Build history of the part. All positions in model axes, mm. A direction names the side the tool comes from. Round coordinates to 2 decimals unless told otherwise and drop trailing zeros. Write each loop counter-clockwise with the first axis right and the second up, starting at its lowest first coordinate (ties: lowest second). Pieces come first, ordered by that corner, then holes.
Item 1: Band-saw the part on A-A, the plane x = 226. Write the cut outline in (y, z).
Item 2: Drop flat-ended pins along their axis: pin 1 Ø2 at (y, z) = (152.5, 74) entering from +X; pin 2 Ø5 at (x, z) = (255.5, 34.5) entering from -Y; pin 3 Ø5 at (x, z) = (257, 33) entering from +Y. Give the stop position or say it passes through.
Item 3: Band-saw the part on D-D, the plane y = 128.5. Write the cut outline in (x, z), then the cut area to 3 significant figures.
Item 4: Wall check: probe 1 along X at (y, z) = (92.5, 76); probe 2 along Y at (x, z) = (237.5, 63); probe 3 along X at (y, z) = (147, 58). Give the ranges that are in metal, low to high.
Item 5: 3-axis set-ups, long thin cutter, end or side, ignore diameter. For faces 1 (the flat face through (256, 102.8, 49)), 2 (the flat face through (234, 82.8, 49)), 3 (the cylindrical face through (214.423, 88.583, 49.3)): which of +Z, -Z, +X, -X, +Y, -Y reach the whole face in a straight line?
Item 6: Band-saw the part on C-C, the plane z = 15. Write the cut outline in (x, y).
Item 7: Mould opens along X. For faces 4 (the flat face through (208.57, 133, 49)), 5 (the cylindrical face through (214.353, 176.946, 49.3)), 6 (the flat face through (256, 162.8, 49)) say: +X half, -X half, draft (parallel to the pull), parting line (faces both ways), or undercut.
Item 8: Band-saw the part on B-B, the plane y = 94. Write the cut outline in (x, z), then the cut area to 3 significant figures.
Autodesk Fusion 360 part; units mm, degrees
sketch "スケッチ1" plane through (0, 0, 0) normal (0, 0, 1) x (1, 0, 0)
  line L0 (213.0702, 173.7996) -> (213.0702, 91.7996)
  line L1 (208.5702, 173.7996) -> (208.5702, 91.7996)
  arc A0 (249.5702, 82.7996) -> (258.5702, 91.7996) centre (249.5702, 91.7996) ccw
  arc A1 (249.5702, 87.2996) -> (254.0702, 91.7996) centre (249.5702, 91.7996) ccw
  line L2 (249.5702, 82.7996) -> (217.5702, 82.7996)
  line L3 (217.5702, 87.2996) -> (249.5702, 87.2996)
  arc A2 (208.5702, 91.7996) -> (217.5702, 82.7996) centre (217.5702, 91.7996) ccw
  arc A3 (213.0702, 91.7996) -> (217.5702, 87.2996) centre (217.5702, 91.7996) ccw
  line L4 (254.0702, 91.7996) -> (254.0702, 102.7996)
  line L5 (258.5702, 91.7996) -> (258.5702, 102.7996)
  line L6 (258.5702, 102.7996) -> (254.0702, 102.7996)
  arc A4 (258.5702, 173.7996) -> (249.5702, 182.7996) centre (249.5702, 173.7996) ccw
  arc A5 (254.0702, 173.7996) -> (249.5702, 178.2996) centre (249.5702, 173.7996) ccw
  arc A6 (217.5702, 182.7996) -> (208.5702, 173.7996) centre (217.5702, 173.7996) ccw
  arc A7 (217.5702, 178.2996) -> (213.0702, 173.7996) centre (217.5702, 173.7996) ccw
  line L7 (217.5702, 178.2996) -> (249.5702, 178.2996)
  line L8 (217.5702, 182.7996) -> (249.5702, 182.7996)
  line L9 (258.5702, 173.7996) -> (258.5702, 162.7996)
  line L10 (254.0702, 173.7996) -> (254.0702, 162.7996)
  line L11 (254.0702, 162.7996) -> (258.5702, 162.7996)
  point P0 (208.5702, 182.7996)
extrude "押し出し1" add sketch "スケッチ1" along normal blind 100
Results:
1. outline: (82.8, 0) - (87.3, 0) - (87.3, 100) - (82.8, 100) - close; (178.3, 0) - (182.8, 0) - (182.8, 100) - (178.3, 100) - close
2. pin 1: stops at x = 213.07
2. pin 2: stops at y = 83.48
2. pin 3: stops at y = 181.33
3. outline: (208.57, 0) - (213.07, 0) - (213.07, 100) - (208.57, 100) - close
3. area: 450 mm2
4. probe 1: x = 208.57 to 213.07, 254.07 to 258.57
4. probe 2: y = 82.8 to 87.3, 178.3 to 182.8
4. probe 3: x = 208.57 to 213.07
5. face 1: +Z, -Z, +X
5. face 2: +Z, -Z, +X, -X, -Y
5. face 3: +Z, -Z
6. outline: (208.57, 91.8) arc R9 ccw to (217.57, 82.8) - (249.57, 82.8) arc R9 ccw to (258.57, 91.8) - (258.57, 102.8) - (254.07, 102.8) - (254.07, 91.8) arc R4.5 cw to (249.57, 87.3) - (217.57, 87.3) arc R4.5 cw to (213.07, 91.8) - (213.07, 173.8) arc R4.5 cw to (217.57, 178.3) - (249.57, 178.3) arc R4.5 cw to (254.07, 173.8) - (254.07, 162.8) - (258.57, 162.8) - (258.57, 173.8) arc R9 ccw to (249.57, 182.8) - (217.57, 182.8) arc R9 ccw to (208.57, 173.8) - close
7. face 4: -X half
7. face 5: undercut
7. face 6: draft
8. outline: (208.57, 0) - (213.07, 0) - (213.07, 100) - (208.57, 100) - close; (254.07, 0) - (258.57, 0) - (258.57, 100) - (254.07, 100) - close
8. area: 900 mm2
